Drawing for the job (mm, zero at the part's lowest x, y, z). A direction names the side the tool comes from. Round coordinates to 2 decimals unless told otherwise and drop trailing zeros. Write each loop counter-clockwise with the first axis right and the second up, starting at its lowest first coordinate (ties: lowest second). Pieces come first, ordered by that corner, then holes. Notation, with made-up numbers: M 78,-40 L 102,-40 A26 ccw 102,-1 Z; hole C -15,70 d9. An arc over 180 degrees is marked long. Use a Markdown table: item, result. Add a question column.
1) Wall check: probe 1 along Z at (x, y) = (4, 4.5); probe 2 along Y at (x, z) = (7, 13.25); probe 3 along Z at (x, y) = (23, 3.25). Give the ranges that are in metal, low to high.
2) Drop flat-ended pins along their axis: P1, Ø4, axis at x = 20, y = 6.5, coming from the -Z side; P2, Ø6, axis at x = 29, z = 8.5, coming from the +Y side; P3, Ø1.5, axis at x = 27, y = 6.5, coming from the -Z side; P4, Ø2.5, axis at x = 27.78, z = 7.94, coming from the +Y side. Give the stop position or say it passes through.
3) Which spindle directions (+Z, -Z, +X, -X, +Y, -Y) get a long thin tool onto all of the face, cutting with end or side? Do the marked faces 4, 5 and 6. Say none if no direction does.
4) Slice it at B-B on x = 4.5. Write the cut outline in (y, z).
5) Two-plate mould, pull along X, no slides. Class the marked faces 1, 2 and 3: released by +X, released by -X, zero draft, split by the parting line, or undercut.
6) Slice it at C-C on y = 3.75. Write the cut outline in (x, z).
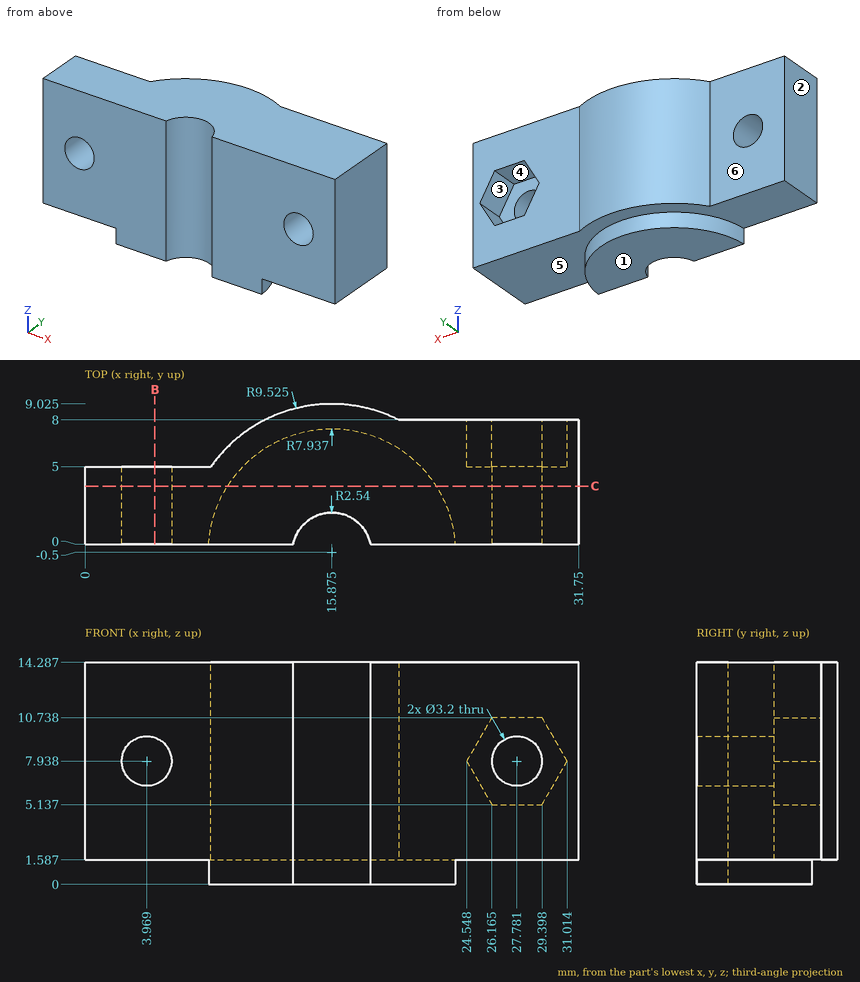
Entries:
| question | item | result |
|---|---|---|
| 1 | probe 1 | z = 1.59 to 6.34, 9.54 to 14.29 |
| 1 | probe 2 | y = 0 to 5 |
| 1 | probe 3 | z = 1.59 to 14.29 |
| 2 | P1 | stops at z = 0 |
| 2 | P2 | stops at y = 8 |
| 2 | P3 | stops at z = 1.59 |
| 2 | P4 | passes through |
| 3 | face 4 | +Y |
| 3 | face 5 | -Z, +Y |
| 3 | face 6 | +Z, -Z, -X, +Y |
| 4 | outline | M 0,1.59 L 5,1.59 L 5,6.43 L 0,6.43 Z; M 0,9.45 L 5,9.45 L 5,14.29 L 0,14.29 Z |
| 5 | face 1 | zero draft |
| 5 | face 2 | released by -X |
| 5 | face 3 | undercut |
| 6 | outline | M 0,1.59 L 9.17,1.59 L 9.17,0 L 22.58,0 L 22.58,1.59 L 31.75,1.59 L 31.75,14.29 L 0,14.29 Z; hole C 3.97,7.94 d3.2; hole C 27.78,7.94 d3.2 |
